Geometry check sheet. Reference: the model listing, model coordinates, mm. Face numbers are marked on the shaded views. A direction names the side the tool comes from. Give positions to 0.01 mm unless a question says otherwise; leave off trailing zeros. Loops run counter-clockwise (first coordinate to the right, second up) from the corner with the lowest first, then second, coordinate; pieces in that order, holes last. Notation, with made-up numbers: (17, 58.25) -> (75, 58.25) arc R21 cw to (75, 71.25) -> close; hole circle Ø1 at (16, 52.5). An arc over 180 degrees is marked (long way). Write each question's results on one line, items separated by ' | '. Start each with the question number.
1) Sectioned sample at C-C on y = 0.6. Record the cut outline in (x, z), then the cut area to 3 significant figures.
2) Depth check by flat-ended pin: pin 1 (1 mm diameter, centred on y = 1.5, z = -3, fed in from -X); pin 2 (1.5 mm diameter, centred on y = 5, z = -4, fed in from -X); pin 3 (3 mm diameter, centred on x = -4.5, z = -3.5, fed in from +Y). Enter the tip coordinate at first touch or a pass-through.
3) Sectioned sample at A-A on z = 0. Record the cut outline in (x, y), then the cut area to 3 significant figures.
4) Sectioned sample at D-D on y = 5.2. Record the cut outline in (x, z).
5) Sectioned sample at B-B on x = 0. Record the cut outline in (y, z), then the cut area to 3 significant figures.
6) Draft check along X on the marked faces 3, 4 and 5. Enter one of: pulls with the +X half, pulls with the -X half, needs draft (parallel to the pull), parting line crosses it, or undercut.
7) Set-up check for the marked faces 1 and 2: record each of +Z, -Z, +X, -X, +Y, -Y from which the full face is reachable in a straight line by a thin tool's end or side.
8) Scan lines: line 1 (X direction, y = 4.2, z = 0); line 2 (X direction, y = 1.9, z = 0); line 3 (Y direction, x = -2.25, z = 2.5). Record each from-to range of solid material in increasing order. Write a range as from..to.
```python
from build123d import *

# Parameters (mm, degrees)
SKETCH1_R           = 6
SKETCH1_R_2         = 3.1
BOSS_EXTRUDE1_DEPTH = 5.8
SKETCH2_R           = 4.1
CUT_EXTRUDE1_DEPTH  = 3.8
CHAMFER1_SIZE       = 1.5


with BuildPart() as part:
    # Sketch1 → Boss-Extrude1 (new body)
    with BuildSketch(Plane(origin=(0, 0, 0), x_dir=(1, 0, 0), z_dir=(0, 1, 0))):
        with Locations(Location((0, 0, 0), (0, 0, 270))):
            Circle(SKETCH1_R)
        with Locations(Location((0, 0, 0), (0, 0, 270))):
            Circle(SKETCH1_R_2, mode=Mode.SUBTRACT)
    extrude(amount=BOSS_EXTRUDE1_DEPTH)

    # Sketch2 → Cut-Extrude1 (cut)
    with BuildSketch(Plane.XZ):
        with Locations(Location((0, 0, 0), (0, 0, 270))):
            Circle(SKETCH2_R)
    extrude(amount=-CUT_EXTRUDE1_DEPTH, mode=Mode.SUBTRACT)

    # Chamfer1
    chamfer1_edges = [part.edges().sort_by_distance(p)[0] for p in [
        (0, 5.8, -6),
    ]]
    chamfer(chamfer1_edges, length=CHAMFER1_SIZE)


solid = part.part
```
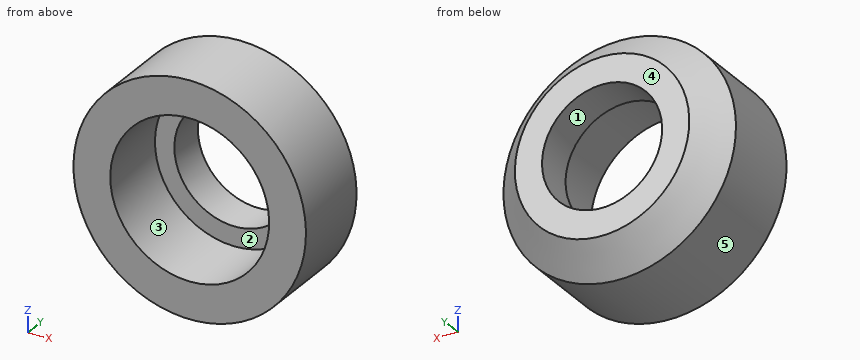
Result:
1) outline: circle Ø12 at (0, 0); hole circle Ø8.2 at (0, 0) | area: 60.3 mm^2
2) pin 1: x = -5.45 | pin 2: x = -4.72 | pin 3: y = 5.8
3) outline: (-6, 0) -> (-4.1, 0) -> (-4.1, 3.8) -> (-3.1, 3.8) -> (-3.1, 5.8) -> (-4.5, 5.8) -> (-6, 4.3) -> close; (3.1, 3.8) -> (4.1, 3.8) -> (4.1, 0) -> (6, 0) -> (6, 4.3) -> (4.5, 5.8) -> (3.1, 5.8) -> close | area: 23.8 mm^2
4) outline: circle Ø10.2 at (0, 0); hole circle Ø6.2 at (0, 0)
5) outline: (0, -6) -> (4.3, -6) -> (5.8, -4.5) -> (5.8, -3.1) -> (3.8, -3.1) -> (3.8, -4.1) -> (0, -4.1) -> close; (0, 4.1) -> (3.8, 4.1) -> (3.8, 3.1) -> (5.8, 3.1) -> (5.8, 4.5) -> (4.3, 6) -> (0, 6) -> close | area: 23.8 mm^2
6) face 3: undercut | face 4: needs draft | face 5: parting line crosses it
7) face 1: +Y, -Y | face 2: -Y
8) line 1: -6..-3.1, 3.1..6 | line 2: -6..-4.1, 4.1..6 | line 3: 3.8..5.8
